Part model, mm, in its own coordinate system. Face numbers are marked on the shaded views. A direction names the side the tool comes from. Round coordinates to 2 decimals unless told otherwise and drop trailing zeros. Loops run counter-clockwise (first coordinate to the right, second up) from the corner with the lowest first, then second, coordinate; pieces in that order, holes last. Notation, with made-up numbers: (81.25, 71.25) - (118.25, 71.25) arc R15 cw to (118.25, 92.25) - close; hole circle Ø7 at (-26.5, 61.25). An arc over 180 degrees is marked (long way). Write each question's results on one line, items separated by ' | '. Start each with the question number.
(1) Cut at C-C, the plane x = 601.5. List the corners of the cut face in (y, z), then the cut area to 3 significant figures.
(2) Cut at B-B, the plane y = 0.2. List the corners of the cut face in (x, z).
(3) Tool access for the marked faces 1 and 2: list every direction of +Z, -Z, +X, -X, +Y, -Y with a clear straight run to the whole face (end or side of a thin tool).
(4) Drill centre lines: L1, parallel to X at y = 1.05, z = 56; L2, parallel to Z at x = 605.25, y = 0.7; L3, parallel to Z at x = 601, y = 1. Where is each one in solid material? Low to high.
(5) Cut at A-A, the plane z = 50.75. List the corners of the cut face in (x, y).
(6) Cut at D-D, the plane x = 603. List the corners of the cut face in (y, z), then the cut area to 3 significant figures.
(7) Flat gauge pins, fed straight in: P1, Ø0.5, axis at y = 1, z = 59.5, coming from the -X side; P2, Ø0.8, axis at x = 599.5, y = 0.5, coming from the +Z side. Where does each tip first touch, or does it go through?
from build123d import *

# Parameters (mm, degrees)
BOSS_EXTRUDE1_DEPTH = 1.6


with BuildPart() as part:
    # Sketch2 → Boss-Extrude1 (new body)
    with BuildSketch(Plane(origin=(0, 0, 0), x_dir=(1, 0, 0), z_dir=(0, 1, 0))):
        with BuildLine():
            Line((606.412306421, -61.448413556), (608.412306421, -61.448413556))
            ThreePointArc((608.412306421, -61.448413556), (608.765859812, -61.301966947), (608.912306421, -60.948413556))
            Line((608.912306421, -60.948413556), (608.912306421, -40.948413556))
            ThreePointArc((608.912306421, -40.948413556), (608.765859812, -40.594860166), (608.412306421, -40.448413556))
            Line((608.412306421, -40.448413556), (599.412306421, -40.448413556))
            ThreePointArc((599.412306421, -40.448413556), (599.05875303, -40.594860166), (598.912306421, -40.948413556))
            Line((598.912306421, -40.948413556), (598.912306421, -58.448413556))
            Line((598.912306421, -58.448413556), (599.662306421, -58.448413556))
            Line((599.662306421, -58.448413556), (599.912306421, -58.448413556))
            Line((599.912306421, -58.448413556), (599.912306421, -48.448413556))
            Line((599.912306421, -48.448413556), (601.912306421, -48.448413556))
            Line((601.912306421, -48.448413556), (601.912306421, -58.448413556))
            Line((601.912306421, -58.448413556), (602.162306421, -58.448413556))
            Line((602.162306421, -58.448413556), (605.912306421, -58.448413556))
            Line((605.912306421, -58.448413556), (605.912306421, -60.948413556))
            ThreePointArc((605.912306421, -60.948413556), (606.05875303, -61.301966947), (606.412306421, -61.448413556))
        make_face()
    extrude(amount=BOSS_EXTRUDE1_DEPTH)


solid = part.part
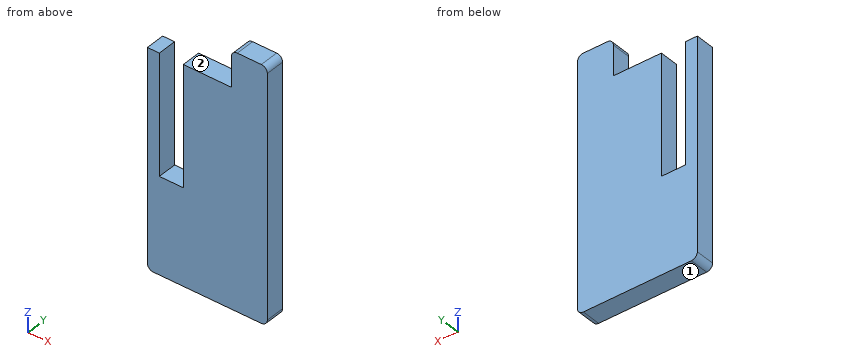
A:
1) outline: (0, 40.45) - (1.6, 40.45) - (1.6, 48.45) - (0, 48.45) - close | area: 12.8 mm2
2) outline: (598.91, 40.95) arc R0.5 ccw to (599.41, 40.45) - (608.41, 40.45) arc R0.5 ccw to (608.91, 40.95) - (608.91, 60.95) arc R0.5 ccw to (608.41, 61.45) - (606.41, 61.45) arc R0.5 ccw to (605.91, 60.95) - (605.91, 58.45) - (601.91, 58.45) - (601.91, 48.45) - (599.91, 48.45) - (599.91, 58.45) - (598.91, 58.45) - close
3) face 1: -Z, +X, -X, +Y, -Y | face 2: +Z, -X, +Y, -Y
4) L1: 598.91 to 599.91, 601.91 to 608.91 | L2: 40.45 to 58.45 | L3: 40.45 to 48.45
5) outline: (598.91, 0) - (599.91, 0) - (599.91, 1.6) - (598.91, 1.6) - close; (601.91, 0) - (608.91, 0) - (608.91, 1.6) - (601.91, 1.6) - close
6) outline: (0, 40.45) - (1.6, 40.45) - (1.6, 58.45) - (0, 58.45) - close | area: 28.8 mm2
7) P1: x = 605.91 | P2: z = 58.45
